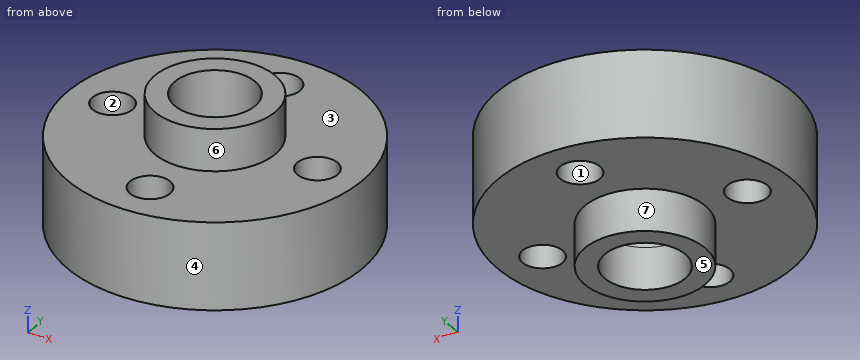
from build123d import *

# Parameters (mm, degrees)
ESQUISSE1_R             = 11
ESQUISSE1_R_2           = 3
EXTRUSION1_DEPTH        = 6.5
ESQUISSE3_R             = 4.5
ESQUISSE3_R_2           = 3
EXTRUSION2_DEPTH        = 3.125
ESQUISSE4_R             = 4.5
ESQUISSE4_R_2           = 3
EXTRUSION3_DEPTH        = 3.125
ENL_V_MAT_EXTRU_1_REACH = 11.625
ESQUISSE5_R             = 1.5


with BuildPart() as part:
    # Esquisse1 → Extrusion1 (new body)
    with BuildSketch(Plane.XY):
        Circle(ESQUISSE1_R)
        Circle(ESQUISSE1_R_2, mode=Mode.SUBTRACT)
    extrude(amount=EXTRUSION1_DEPTH)

    # Esquisse3 → Extrusion2 (add)
    with BuildSketch(Plane.XY.offset(6.5)):
        Circle(ESQUISSE3_R)
        Circle(ESQUISSE3_R_2, mode=Mode.SUBTRACT)
    extrude(amount=EXTRUSION2_DEPTH)

    # Esquisse4 → Extrusion3 (add)
    with BuildSketch(Plane(origin=(0, 0, 0), x_dir=(-1, 0, 0), z_dir=(0, 0, -1))):
        Circle(ESQUISSE4_R)
        Circle(ESQUISSE4_R_2, mode=Mode.SUBTRACT)
    extrude(amount=EXTRUSION3_DEPTH)

    # Esquisse5 → Enlèv. mat.-Extru.1 (cut, up to next)
    with BuildSketch(Plane.XY.offset(6.5), mode=Mode.PRIVATE) as enl_v_mat_extru_1_sk1:
        with Locations((0, 7.75)):
            Circle(ESQUISSE5_R)
    enl_v_mat_extru_1_tool1 = extrude(enl_v_mat_extru_1_sk1.sketch, amount=-ENL_V_MAT_EXTRU_1_REACH, mode=Mode.PRIVATE) & part.part
    add(enl_v_mat_extru_1_tool1.solids().sort_by_distance((0, 7.75, 6.5))[0], mode=Mode.SUBTRACT)
    # Esquisse5 → Enlèv. mat.-Extru.1 (cut, up to next)
    with BuildSketch(Plane.XY.offset(6.5), mode=Mode.PRIVATE) as enl_v_mat_extru_1_sk2:
        with Locations((0, -7.75)):
            Circle(ESQUISSE5_R)
    enl_v_mat_extru_1_tool2 = extrude(enl_v_mat_extru_1_sk2.sketch, amount=-ENL_V_MAT_EXTRU_1_REACH, mode=Mode.PRIVATE) & part.part
    add(enl_v_mat_extru_1_tool2.solids().sort_by_distance((0, -7.75, 6.5))[0], mode=Mode.SUBTRACT)
    # Esquisse5 → Enlèv. mat.-Extru.1 (cut, up to next)
    with BuildSketch(Plane.XY.offset(6.5), mode=Mode.PRIVATE) as enl_v_mat_extru_1_sk3:
        with Locations((-7.75, 0)):
            Circle(ESQUISSE5_R)
    enl_v_mat_extru_1_tool3 = extrude(enl_v_mat_extru_1_sk3.sketch, amount=-ENL_V_MAT_EXTRU_1_REACH, mode=Mode.PRIVATE) & part.part
    add(enl_v_mat_extru_1_tool3.solids().sort_by_distance((-7.75, 0, 6.5))[0], mode=Mode.SUBTRACT)
    # Esquisse5 → Enlèv. mat.-Extru.1 (cut, up to next)
    with BuildSketch(Plane.XY.offset(6.5), mode=Mode.PRIVATE) as enl_v_mat_extru_1_sk4:
        with Locations((7.75, 0)):
            Circle(ESQUISSE5_R)
    enl_v_mat_extru_1_tool4 = extrude(enl_v_mat_extru_1_sk4.sketch, amount=-ENL_V_MAT_EXTRU_1_REACH, mode=Mode.PRIVATE) & part.part
    add(enl_v_mat_extru_1_tool4.solids().sort_by_distance((7.75, 0, 6.5))[0], mode=Mode.SUBTRACT)


solid = part.part
Geometry: final body of the model. Coordinates: model frame, mm. Face numbers are marked on the shaded views. A direction names the side the tool comes from. Give positions to 0.01 mm unless a question says otherwise; leave off trailing zeros. Loops run counter-clockwise (first coordinate to the right, second up) from the corner with the lowest first, then second, coordinate; pieces in that order, holes last. Notation, with made-up numbers: (10, -28.5) -> (66, -28.5) arc R17 cw to (66, -13.5) -> close; hole circle Ø2 at (17.5, 5). An arc over 180 degrees is marked (long way). Put each result on its own line as item: value.
1. Pin query (flat end, axial travel): P1, Ø5, axis at x = 0, y = 0, coming from the +Z side; P2, Ø1, axis at x = -5, z = 4.5, coming from the +Y side; P3, Ø3.5, axis at x = 7.75, y = 0, coming from the +Z side; P4, Ø5, axis at x = 0, y = -7.75, coming from the -Z side. Return the tip coordinate at first contact, or that it passes through.
Taken from the geometry:
P1: passes through
P2: stops at y = 10.04
P3: stops at z = 6.5
P4: stops at z = 0
2. Cut plane A-A (x = 0). Return the cut outline in (y, z) (3 decimals), plus the area to 4 significant figures.
Taken from the geometry:
outline: (-11, 0) -> (-9.25, 0) -> (-9.25, 6.5) -> (-11, 6.5) -> close; (-6.25, 0) -> (-4.5, 0) -> (-4.5, -3.125) -> (-3, -3.125) -> (-3, 9.625) -> (-4.5, 9.625) -> (-4.5, 6.5) -> (-6.25, 6.5) -> close; (3, -3.125) -> (4.5, -3.125) -> (4.5, 0) -> (6.25, 0) -> (6.25, 6.5) -> (4.5, 6.5) -> (4.5, 9.625) -> (3, 9.625) -> close; (9.25, 0) -> (11, 0) -> (11, 6.5) -> (9.25, 6.5) -> close
area: 83.75 mm2
3. Cut plane C-C (z = 0.5). Return the cut outline in (x, y).
Taken from the geometry:
outline: circle Ø22 at (0, 0); hole circle Ø3 at (-7.75, 0); hole circle Ø6 at (0, 0); hole circle Ø3 at (0, -7.75); hole circle Ø3 at (0, 7.75); hole circle Ø3 at (7.75, 0)
4. Cut plane D-D (y = -7.75). Return the cut outline in (x, z), plus the area to 3 significant figures.
Taken from the geometry:
outline: (-7.81, 0) -> (-1.5, 0) -> (-1.5, 6.5) -> (-7.81, 6.5) -> close; (1.5, 0) -> (7.81, 0) -> (7.81, 6.5) -> (1.5, 6.5) -> close
area: 82.0 mm2
5. Set-up query: the marked faces 5, 6 and 7. Return all of +Z, -Z, +X, -X, +Y, -Y with unobstructed straight access to the full face (end or side cutting, diameter ignored); none if empty.
Taken from the geometry:
face 5: -Z, +X, -X, +Y, -Y
face 6: +Z
face 7: -Z
6. Ray query, line 1 along Y through (x, z) = (0, 4); line 2 along Y through (x, z) = (0, -0.85); line 3 along Z through (x, y) = (-10, 1). Return the intervals inside material, ascending. Write a range as [from, to].
Taken from the geometry:
line 1: y = [-11, -9.25], [-6.25, -3], [3, 6.25], [9.25, 11]
line 2: y = [-4.5, -3], [3, 4.5]
line 3: z = [0, 6.5]
7. Pull-direction query (Y, two-part tool) for the marked faces 1, 2, 3 and 4; classes: released by +Y, released by -Y, zero draft, split by the parting line, or undercut.
Taken from the geometry:
face 1: undercut
face 2: undercut
face 3: zero draft
face 4: split by the parting line
